```python
from build123d import *

# Parameters (mm, degrees)
SKETCH1_W           = 260.35
SKETCH1_H           = 159.592906802
BOSS_EXTRUDE1_DEPTH = 3.175
SKETCH2_W           = 3.175
SKETCH2_H           = 26.5988178
CUT_EXTRUDE1_DEPTH  = 6.35
LPATTERN1_COUNT     = 3
LPATTERN1_PITCH     = 53.19763554
SKETCH3_W           = 3.175
SKETCH3_H           = 26.59881777
CUT_EXTRUDE3_DEPTH  = 6.35
LPATTERN3_COUNT     = 3
LPATTERN3_PITCH     = 53.19763554
SKETCH5_W           = 3.175
SKETCH5_H           = 3
CUT_EXTRUDE4_DEPTH  = 12
SKETCH6_W           = 2.2
SKETCH6_H           = 3.175
CUT_EXTRUDE5_DEPTH  = 1
SKETCH8_W           = 2.2
SKETCH8_H           = 3.175
CUT_EXTRUDE6_DEPTH  = 1
LPATTERN5_COUNT     = 3
LPATTERN5_PITCH     = 53.34
SKETCH9_W           = 3.175
SKETCH9_H           = 3
CUT_EXTRUDE7_DEPTH  = 12
SKETCH10_W          = 2.2
SKETCH10_H          = 3.175
CUT_EXTRUDE8_DEPTH  = 1
SKETCH11_W          = 2.2
SKETCH11_H          = 3.175
CUT_EXTRUDE9_DEPTH  = 1
LPATTERN6_COUNT     = 3
LPATTERN6_PITCH     = 53.34
CUT_EXTRUDE10_DEPTH = 153.718974674
LPATTERN7_COUNT     = 2
LPATTERN7_PITCH     = 53.34
LPATTERN8_COUNT     = 2
LPATTERN8_PITCH     = 53.34
SKETCH15_W          = 12.7
SKETCH15_H          = 3.175
BOSS_EXTRUDE2_DEPTH = 9.144
SKETCH16_W          = 25.4
SKETCH16_H          = 3.175
BOSS_EXTRUDE3_DEPTH = 6.35
LPATTERN9_COUNT     = 2
LPATTERN9_PITCH     = 53.34
LPATTERN10_COUNT    = 2
LPATTERN10_PITCH    = 53.34


with BuildPart() as part:
    # Sketch1 → Boss-Extrude1 (new body)
    with BuildSketch(Plane.XY):
        Rectangle(SKETCH1_W, SKETCH1_H)
    extrude(amount=BOSS_EXTRUDE1_DEPTH)

    # Sketch2 → Cut-Extrude1 (cut)
    with BuildSketch(Plane.ZY.offset(130.175)):
        with Locations((1.5875, 66.497044501)):
            Rectangle(SKETCH2_W, SKETCH2_H)
    cut_extrude1 = extrude(amount=-CUT_EXTRUDE1_DEPTH, mode=Mode.SUBTRACT)

    # LPattern1: Cut-Extrude1 ×3
    with Locations(*[(0, -i * LPATTERN1_PITCH, 0) for i in range(1, LPATTERN1_COUNT)]):
        add(cut_extrude1, mode=Mode.SUBTRACT)

    # Sketch3 → Cut-Extrude3 (cut)
    with BuildSketch(Plane(origin=(130.175, 0, 0), x_dir=(0, 0, -1), z_dir=(1, 0, 0))):
        with Locations((-1.5875, -39.898226818)):
            Rectangle(SKETCH3_W, SKETCH3_H)
    cut_extrude3 = extrude(amount=-CUT_EXTRUDE3_DEPTH, mode=Mode.SUBTRACT)

    # LPattern3: Cut-Extrude3 ×3
    with Locations(*[(0, i * LPATTERN3_PITCH, 0) for i in range(1, LPATTERN3_COUNT)]):
        add(cut_extrude3, mode=Mode.SUBTRACT)

    # Sketch5 → Cut-Extrude4 (cut)
    with BuildSketch(Plane.ZY.offset(123.825)):
        with Locations((1.5875, -39.898226579)):
            Rectangle(SKETCH5_W, SKETCH5_H)
    cut_extrude4 = extrude(amount=-CUT_EXTRUDE4_DEPTH, mode=Mode.SUBTRACT)

    # Sketch6 → Cut-Extrude5 (cut)
    with BuildSketch(Plane.XZ.offset(38.398226579)):
        with Locations((-117.925, 1.5875)):
            Rectangle(SKETCH6_W, SKETCH6_H)
    cut_extrude5 = extrude(amount=-CUT_EXTRUDE5_DEPTH, mode=Mode.SUBTRACT)

    # Sketch8 → Cut-Extrude6 (cut)
    with BuildSketch(Plane(origin=(0, -41.398226579, 0), x_dir=(1, 0, 0), z_dir=(0, 1, 0))):
        with Locations((-117.925, -1.5875)):
            Rectangle(SKETCH8_W, SKETCH8_H)
    cut_extrude6 = extrude(amount=-CUT_EXTRUDE6_DEPTH, mode=Mode.SUBTRACT)

    # LPattern5: Cut-Extrude4, Cut-Extrude5, Cut-Extrude6 ×3
    with Locations(*[(0, i * LPATTERN5_PITCH, 0) for i in range(1, LPATTERN5_COUNT)]):
        add(cut_extrude4, mode=Mode.SUBTRACT)
        add(cut_extrude5, mode=Mode.SUBTRACT)
        add(cut_extrude6, mode=Mode.SUBTRACT)

    # Sketch9 → Cut-Extrude7 (cut)
    with BuildSketch(Plane(origin=(123.825, 0, 0), x_dir=(0, 0, -1), z_dir=(1, 0, 0))):
        with Locations((-1.5875, -39.898226818)):
            Rectangle(SKETCH9_W, SKETCH9_H)
    cut_extrude7 = extrude(amount=-CUT_EXTRUDE7_DEPTH, mode=Mode.SUBTRACT)

    # Sketch10 → Cut-Extrude8 (cut)
    with BuildSketch(Plane.XZ.offset(38.398226818)):
        with Locations((117.925, 1.5875)):
            Rectangle(SKETCH10_W, SKETCH10_H)
    cut_extrude8 = extrude(amount=-CUT_EXTRUDE8_DEPTH, mode=Mode.SUBTRACT)

    # Sketch11 → Cut-Extrude9 (cut)
    with BuildSketch(Plane(origin=(0, -41.398226818, 0), x_dir=(1, 0, 0), z_dir=(0, 1, 0))):
        with Locations((117.925, -1.5875)):
            Rectangle(SKETCH11_W, SKETCH11_H)
    cut_extrude9 = extrude(amount=-CUT_EXTRUDE9_DEPTH, mode=Mode.SUBTRACT)

    # LPattern6: Cut-Extrude7, Cut-Extrude8, Cut-Extrude9 ×3
    with Locations(*[(0, i * LPATTERN6_PITCH, 0) for i in range(1, LPATTERN6_COUNT)]):
        add(cut_extrude7, mode=Mode.SUBTRACT)
        add(cut_extrude8, mode=Mode.SUBTRACT)
        add(cut_extrude9, mode=Mode.SUBTRACT)

    # Sketch4 → Cut-Extrude10 (cut, through all)
    with BuildSketch(Plane.XY.offset(3.175)):
        Polygon((-6.35, -79.796453401), (-6.35, -70.685115582), (-12.899606221, -70.685115582), (-12.899606221, -64.335115582), (12.500393779, -64.335115582), (12.500393779, -70.685115582), (6.35, -70.685115582), (6.35, -79.796453401), align=None)
    cut_extrude10 = extrude(amount=-CUT_EXTRUDE10_DEPTH, mode=Mode.SUBTRACT)

    # LPattern7: Cut-Extrude10 ×2
    with Locations(*[(-i * LPATTERN7_PITCH, 0, 0) for i in range(1, LPATTERN7_COUNT)]):
        add(cut_extrude10, mode=Mode.SUBTRACT)

    # LPattern8: Cut-Extrude10 ×2
    with Locations(*[(i * LPATTERN8_PITCH, 0, 0) for i in range(1, LPATTERN8_COUNT)]):
        add(cut_extrude10, mode=Mode.SUBTRACT)

    # Sketch15 → Boss-Extrude2 (add)
    with BuildSketch(Plane(origin=(0, 79.796453401, 0), x_dir=(1, 0, 0), z_dir=(0, 1, 0))):
        with Locations((0, -1.5875)):
            Rectangle(SKETCH15_W, SKETCH15_H)
    boss_extrude2 = extrude(amount=BOSS_EXTRUDE2_DEPTH)

    # Sketch16 → Boss-Extrude3 (add)
    with BuildSketch(Plane(origin=(0, 88.940453401, 0), x_dir=(1, 0, 0), z_dir=(0, 1, 0))):
        with Locations((0, -1.5875)):
            Rectangle(SKETCH16_W, SKETCH16_H)
    boss_extrude3 = extrude(amount=BOSS_EXTRUDE3_DEPTH)

    # LPattern9: Boss-Extrude2, Boss-Extrude3 ×2
    with Locations(*[(i * LPATTERN9_PITCH, 0, 0) for i in range(1, LPATTERN9_COUNT)]):
        add(boss_extrude2)
        add(boss_extrude3)

    # LPattern10: Boss-Extrude2, Boss-Extrude3 ×2
    with Locations(*[(-i * LPATTERN10_PITCH, 0, 0) for i in range(1, LPATTERN10_COUNT)]):
        add(boss_extrude2)
        add(boss_extrude3)


solid = part.part
```
Input: part model. Units: mm. Frame: model coordinates. Round coordinates to 2 decimals unless told otherwise and drop trailing zeros. Loops run counter-clockwise (first coordinate to the right, second up) from the corner with the lowest first, then second, coordinate; pieces in that order, holes last. Notation, with made-up numbers: (86, 17.25) - (91, 17.25) arc R17 cw to (91, 27.25) - close; hole circle Ø4 at (87, -32.75). An arc over 180 degrees is marked (long way). One line per item, written item: value. Start each with the question number.
(1) Section A-A, the plane y = -67. Return loops of the section in (x, z) (3 decimals).
(2) Section B-B, the plane x = -16. Return loops of the section in (y, z) (3 decimals), plus the area to 3 significant figures.
(3) Contact query for flat-ended pins moving along their axis: P1, Ø0.5, axis at y = 65, z = 1.5, coming from the +X side (3 decimals); P2, Ø1, axis at x = 2, z = 2.5, coming from the -Y side; P3, Ø1.5, axis at y = -40, z = 2, coming from the +X side (3 decimals). Output: stop coordinate, or through.
(4) Ray query, line 1 (X direction, y = -65.5, z = 0.35) (3 decimals); line 2 (X direction, y = 81, z = 1.65); line 3 (X direction, y = -71.5, z = 0.9) (3 decimals). Return the intervals inside material, ascending. Write a range as [from, to].
(5) Section C-C, the plane y = -32. Return loops of the section in (x, z) (3 decimals), plus the area to 3 significant figures.
Results below:
1. outline: (-130.175, 0) - (-66.24, 0) - (-66.24, 3.175) - (-130.175, 3.175) - close; (-40.84, 0) - (-12.9, 0) - (-12.9, 3.175) - (-40.84, 3.175) - close; (12.5, 0) - (40.44, 0) - (40.44, 3.175) - (12.5, 3.175) - close; (65.84, 0) - (130.175, 0) - (130.175, 3.175) - (65.84, 3.175) - close
2. outline: (-79.796, 0) - (79.796, 0) - (79.796, 3.175) - (-79.796, 3.175) - close
2. area: 507 mm^2
3. P1: x = 123.825
3. P2: y = -64.34
3. P3: x = 111.825
4. line 1: [-130.175, -66.24], [-40.84, -12.9], [12.5, 40.44], [65.84, 130.175]
4. line 2: [-59.69, -46.99], [-6.35, 6.35], [46.99, 59.69]
4. line 3: [-130.175, -59.69], [-46.99, -6.35], [6.35, 46.99], [59.69, 130.175]
5. outline: (-123.825, 0) - (123.825, 0) - (123.825, 3.175) - (-123.825, 3.175) - close
5. area: 786 mm^2
